Here's the drawing with two shaded views (mm, measured from the low corner). I have some questions. Coordinates: 2 decimals unless noted, no trailing zeros. Order: outer loops, then holes, each group sorted by start corner. A loop starts at its lowest first (then second) coordinate and runs counter-clockwise, first axis right, second up. Notation, with made-up numbers: (3, 47.5) -> (32, 47.5) arc R19 cw to (32, 72.5) -> close; hole circle Ø4 at (69, 76). An arc over 180 degrees is marked (long way). Return JSON: item names as keys, results as strings. Group by question number.
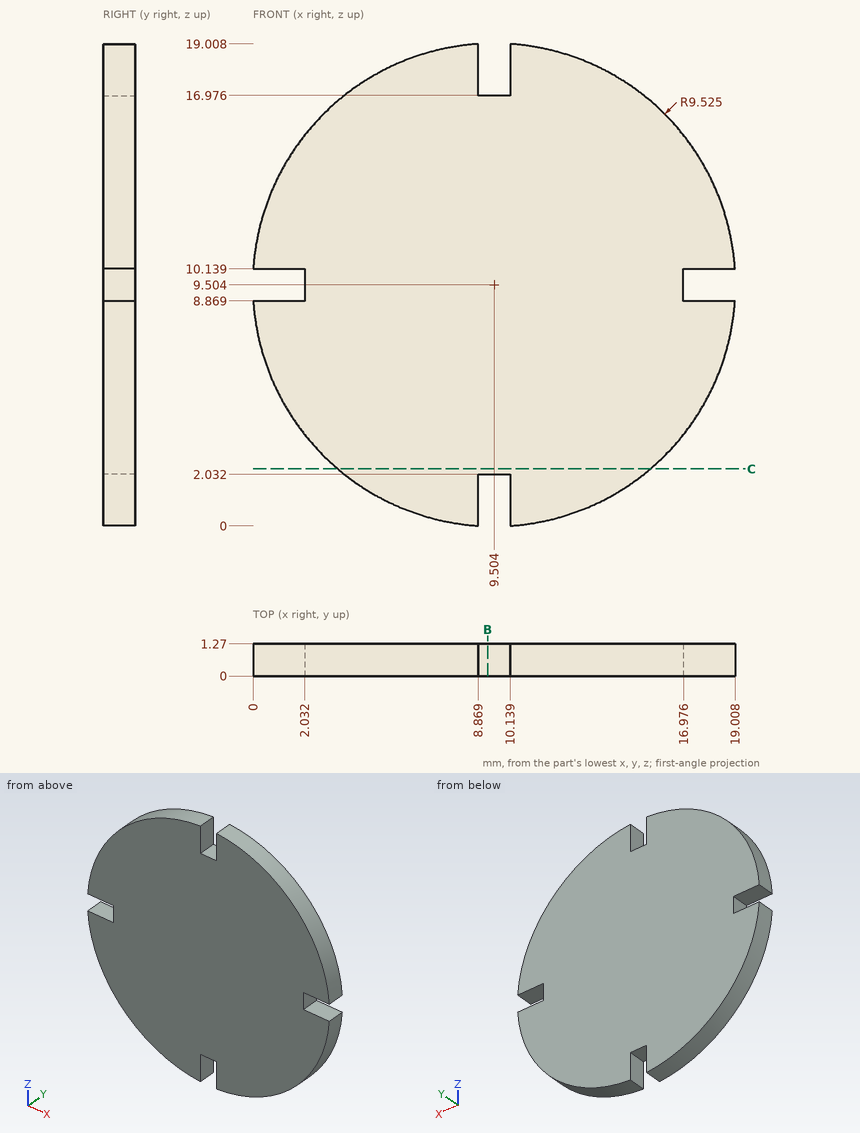
Q1. I want a section at C-C on z = 2.25. Please give me the cut outline in (x, y), and give its area (3 significant figures).
Q2. I need wall thicknesses on line 1 along Z through (x, y) = (1.5, 0.85) (1 decimal); line 2 along X through (y, z) = (0.2, 17.5); line 3 along X through (y, z) = (0.45, 18.25) (1 decimal). Which ranges of each line are inside material? Lowest first, please. Write a range as from..to.
Q3. I want a section at B-B on x = 9.25. Please give me the cut outline in (y, z) (1 decimal), and give its area (3 significant figures).
Response values:
{
 "1": {"outline": "(3.33, 0) -> (15.68, 0) -> (15.68, 1.27) -> (3.33, 1.27) -> close", "area": "15.7 mm²"},
 "2": {"line 1": "z = 4.3..8.9, 10.1..14.7", "line 2": "x = 4.33..8.87, 10.14..14.68", "line 3": "x = 5.7..8.9, 10.1..13.3"},
 "3": {"outline": "(0, 2) -> (1.3, 2) -> (1.3, 17) -> (0, 17) -> close", "area": "19.0 mm²"}
}
